Verification items for the finished model (mm, model axes). Face numbers are marked on the shaded views. A direction names the side the tool comes from. Round coordinates to 2 decimals unless told otherwise and drop trailing zeros. Write each loop counter-clockwise with the first axis right and the second up, starting at its lowest first coordinate (ties: lowest second). Pieces come first, ordered by that corner, then holes.
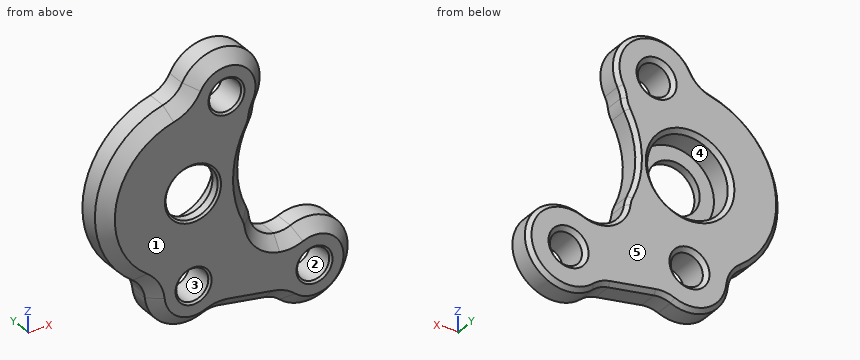
from build123d import *

# Parameters (mm, degrees)
SKETCH1_R           = 9
SKETCH1_R_2         = 4.025
BOSS_EXTRUDE1_DEPTH = 3.5
SKETCH2_R           = 4.1
SKETCH2_R_2         = 1.6
BOSS_EXTRUDE2_DEPTH = 3.5
SKETCH6_R           = 9
CUT_EXTRUDE2_DEPTH  = 17.27435259
CUT_EXTRUDE1_START  = -3.5
SKETCH3_R           = 1.6
CUT_EXTRUDE1_DEPTH  = 3.5
SKETCH4_R           = 1.6
BOSS_EXTRUDE3_DEPTH = 3.5
SKETCH5_R           = 4.025
SKETCH5_R_2         = 2.6
BOSS_EXTRUDE4_DEPTH = 1
FILLET1_R           = 3
FILLET9_R           = 3
CHAMFER_1_SIZE      = 1.2
CHAMFER_2_SIZE      = 0.2
CHAMFER_3_SIZE      = 0.4


with BuildPart() as part:
    # Sketch1 → Boss-Extrude1 (new body)
    with BuildSketch(Plane(origin=(0, 0, 0), x_dir=(1, 0, 0), z_dir=(0, 1, 0))):
        with Locations(Location((0, 0, 0), (0, 0, 270))):
            Circle(SKETCH1_R)
        with Locations(Location((0, 0, 0), (0, 0, 270))):
            Circle(SKETCH1_R_2, mode=Mode.SUBTRACT)
    extrude(amount=BOSS_EXTRUDE1_DEPTH)

    # Sketch2 → Boss-Extrude2 (add)
    # profile 1 of 2: a face of its own
    with BuildSketch(Plane(origin=(0, 3.5, 0), x_dir=(1, 0, 0), z_dir=(0, 1, 0))):
        with Locations((3.343277014, -8.355985807)):
            Circle(SKETCH2_R)
        with Locations((3.343277014, -8.355985807)):
            Circle(SKETCH2_R_2, mode=Mode.SUBTRACT)
    # profile 2 of 2: a face of its own
    with BuildSketch(Plane(origin=(0, 3.5, 0), x_dir=(1, 0, 0), z_dir=(0, 1, 0))):
        with Locations((0.061177946, 8.999792068)):
            Circle(SKETCH2_R)
        with Locations((0.061177946, 8.999792068)):
            Circle(SKETCH2_R_2, mode=Mode.SUBTRACT)
    extrude(amount=-BOSS_EXTRUDE2_DEPTH)

    # Sketch6 → Cut-Extrude2 (cut, through all)
    with BuildSketch(Plane(origin=(0, 0, 0), x_dir=(-1, 0, 0), z_dir=(0, -1, 0))):
        with Locations((-14.2, 0)):
            Circle(SKETCH6_R)
    extrude(amount=-CUT_EXTRUDE2_DEPTH, mode=Mode.SUBTRACT)

    # Sketch3 → Cut-Extrude1 (cut)
    with BuildSketch(Plane(origin=(0, 0, 0), x_dir=(-1, 0, 0), z_dir=(0, -1, 0)).offset(CUT_EXTRUDE1_START)):
        with Locations(Location((-0.061177946, 8.999792068, 0), (0, 0, 270))):
            Circle(SKETCH3_R)
        with Locations(Location((-3.343277014, -8.355985807, 0), (0, 0, 270))):
            Circle(SKETCH3_R)
    extrude(amount=CUT_EXTRUDE1_DEPTH, mode=Mode.SUBTRACT)

    # Sketch4 → Boss-Extrude3 (add)
    with BuildSketch(Plane(origin=(0, 0, 0), x_dir=(-1, 0, 0), z_dir=(0, -1, 0))):
        with BuildLine():
            Line((-2.353733001, 12.398937743), (-8.897987933, 13.432234974))
            ThreePointArc((-8.897987933, 13.432234974), (-16.176141716, 11.544244815), (-9.833757914, 7.505656319))
            Line((-9.833757914, 7.505656319), (-5.813078926, 6.870816065))
            ThreePointArc((-5.813078926, 6.870816065), (-4.964487715, 7.506920922), (-4.04696144, 8.038787415))
            ThreePointArc((-4.04696144, 8.038787415), (-3.883103044, 10.484005175), (-2.353733001, 12.398937743))
        make_face()
        with Locations(Location((-12.126312969, 10.904801994, 0), (0, 0, 90))):
            Circle(SKETCH4_R, mode=Mode.SUBTRACT)
    extrude(amount=-BOSS_EXTRUDE3_DEPTH)

    # Sketch5 → Boss-Extrude4 (add)
    with BuildSketch(Plane(origin=(0, 0, 0), x_dir=(-1, 0, 0), z_dir=(0, -1, 0))):
        with Locations(Location((0, 0, 0), (0, 0, 90))):
            Circle(SKETCH5_R)
        with Locations(Location((0, 0, 0), (0, 0, 90))):
            Circle(SKETCH5_R_2, mode=Mode.SUBTRACT)
    extrude(amount=-BOSS_EXTRUDE4_DEPTH)

    # Fillet1
    # the kernel refuses this fillet: 3 mm, written as the material it adds along each edge
    with BuildSketch(Plane(origin=(-0.71019136, 3.5, 8.97193559), x_dir=(-0.9865858542334134, 0, -0.1632432302624714), z_dir=(0, -1, 0))) as fillet1_piece_1:
        with BuildLine():
            CenterArc((1.782533661, -2.98917289), FILLET1_R, 94.869271374, 48.27534012)
            ThreePointArc((-0.617922081, -1.189780705), (-0.260000299, -0.620318503), (0, 0))
            ThreePointArc((0, 0), (0.763942997, -0.03248133), (1.527885995, 0))
        make_face()
    extrude(amount=3.5)
    with BuildSketch(Plane(origin=(-3.93730186, 3.5, -8.093062095), x_dir=(-0.8588495215516518, 0, 0.5122279759350309), z_dir=(0, -1, 0))) as fillet1_piece_2:
        with BuildLine():
            CenterArc((1.782533661, 2.98917289), FILLET1_R, 216.855388506, 48.27534012)
            ThreePointArc((-0.617922081, 1.189780705), (-0.260000299, 0.620318503), (0, 0))
            ThreePointArc((0, 0), (0.763942997, 0.03248133), (1.527885995, 0))
        make_face()
    extrude(amount=3.5)
    with BuildSketch(Plane(origin=(8.897987933, 0, -13.432234974), x_dir=(-0.9877631090139599, 0, 0.15596166346598195), z_dir=(0, 1, 0))) as fillet1_piece_3:
        with BuildLine():
            CenterArc((1.001412857, -3), FILLET1_R, 90, 32.320518146)
            ThreePointArc((-0.602552177, -0.464788732), (-0.290469322, -0.24640426), (0, 0))
            Line((0, 0), (1.001412857, 0))
        make_face()
    extrude(amount=3.5)
    with BuildSketch(Plane(origin=(2.353733001, 0, -12.398937743), x_dir=(-0.8773738132879287, 0, -0.4798074527939294), z_dir=(0, 1, 0)), Plane(origin=(9.833757914, 0, -7.505656319), x_dir=(0.8773738132879222, 0, 0.47980745279394127), z_dir=(0, 1, 0))) as fillet1_piece_4:
        with BuildLine():
            CenterArc((1.039393717, -2.987053466), FILLET1_R, 95.324882893, 32.320518146)
            Line((-0.792924625, -0.611635715), (0, 0))
            ThreePointArc((0, 0), (0.380492343, -0.017693596), (0.760984685, 0))
        make_face()
    extrude(amount=3.5)
    # the kernel refuses this fillet: 3 mm, written as the material it takes off along each edge
    with BuildSketch(Plane(origin=(7.1, 6.983871428, 5.530822724), x_dir=(-0.6413091964506672, 0, 0.7672825519636162), z_dir=(0, -1, 0))) as fillet1_2_piece_1:
        with BuildLine():
            CenterArc((2.400494629, 2.413903277), FILLET1_R, 201.072777054, 32.502187501)
            ThreePointArc((-0.398878795, 1.335242797), (-0.173557144, 0.675353237), (0, 0))
            ThreePointArc((0, 0), (0.309591521, -0.005326404), (0.619183042, 0))
        make_face()
    extrude(amount=10.467742856, mode=Mode.SUBTRACT)
    with BuildSketch(Plane(origin=(7.1, 8.410224582, -5.530822724), x_dir=(-0.5247859915025788, 0, 0.8512341999254115), z_dir=(0, -1, 0))) as fillet1_2_piece_2:
        with BuildLine():
            CenterArc((2.291438138, 2.982087035), FILLET1_R, 203.232841743, 60.502793026)
            ThreePointArc((-0.465290008, 1.798680965), (-0.279182448, 0.88730199), (0, 0))
            ThreePointArc((0, 0), (0.982044916, 0.053738894), (1.964089833, 0))
        make_face()
    extrude(amount=13.320449164, mode=Mode.SUBTRACT)

    # Fillet9
    fillet9_edges = [part.edges().sort_by_distance(p)[0] for p in [
        (6.702912221, 1.75, 6.005911068),
        (5.813078926, 1.75, -6.870816065),
    ]]
    fillet(fillet9_edges, radius=FILLET9_R)

    # 倒角1
    chamfer_1_edges = [part.edges().sort_by_distance(p)[0] for p in [
        (16.176141716, 0, -11.544244815),
        (5.625860467, 0, -12.915586358),
        (-2.007663811, 0, -12.539551069),
        (5.204560758, 0, 0.286483569),
        (5.220072831, 0, 12.001206989),
        (-8.84326494, 0, 1.672323294),
        (6.564091926, 0, 4.905386326),
        (9.687844205, 0, -7.362609827),
        (8.715099113, 0, -13.523365587),
        (2.49964671, 0, -12.541984235),
        (-4.406035705, 0, -8.239061366),
        (-1.093245074, 0, 9.27901385),
        (8.843752485, 0, -7.349340608),
        (6.238006504, 0, -4.301725459),
        (7.158194759, 0, -6.475494242),
        (6.796639749, 0, 5.998875214),
    ]]
    chamfer(chamfer_1_edges, length=CHAMFER_1_SIZE)

    # 倒角2
    chamfer_2_edges = [part.edges().sort_by_distance(p)[0] for p in [
        (4.706817353, 0, 9.19309855),
        (1.13707684, 0, -7.815544808),
        (12.126312969, 0, -9.304801994),
        (0, 0, 2.6),
    ]]
    chamfer(chamfer_2_edges, length=CHAMFER_2_SIZE)

    # 倒角3
    chamfer_3_edges = [part.edges().sort_by_distance(p)[0] for p in [
        (16.176141716, 3.5, -11.544244815),
        (5.625860467, 3.5, -12.915586358),
        (-2.007663811, 3.5, -12.539551069),
        (5.204560758, 3.5, 0.286483569),
        (-8.84326494, 3.5, 1.672323294),
        (5.220072831, 3.5, 12.001206989),
        (6.238006504, 3.5, -4.301725459),
        (9.687844205, 3.5, -7.362609827),
        (8.715099113, 3.5, -13.523365587),
        (2.49964671, 3.5, -12.541984235),
        (-4.406035705, 3.5, -8.239061366),
        (-1.093245074, 3.5, 9.27901385),
        (8.843752485, 3.5, -7.349340608),
        (6.564091926, 3.5, 4.905386326),
        (7.158194759, 3.5, -6.475494242),
        (6.796639749, 3.5, 5.998875214),
        (4.706817353, 3.5, 9.19309855),
        (1.13707684, 3.5, -7.815544808),
        (0, 3.5, -4.025),
        (12.126312969, 3.5, -9.304801994),
    ]]
    chamfer(chamfer_3_edges, length=CHAMFER_3_SIZE)


solid = part.part
Q1. Tool access check on the marked faces 4 and 5. Record the directions out of +Z, -Z, +X, -X, +Y, -Y that give a thin tool (end or side, any length) a straight path to the whole face; none if there is none.
Recorded:
face 4: +Y
face 5: +Z, -Z, +X, -X, +Y
Q2. Sectioned sample at B-B (z = -10). Give the number of separate pieces and of enclosed holes in the cut face, plus the area to 3 significant figures.
Recorded:
separate pieces: 3
enclosed holes: 0
area: 50.0 mm2
Q3. Release check for a two-part mould opening along Z. For the marked faces 1, 2 and 3 record: released by +Z, released by -Z, zero draft, split by the parting line, or undercut.
Recorded:
face 1: zero draft
face 2: undercut
face 3: undercut
Q4. Depth check by flat-ended pin: P1, Ø2.5, axis at x = 0.06, z = -9, coming from the -Y side. Enter the tip coordinate at first touch or a pass-through.
Recorded:
P1: passes through
Q5. Material ranges on line 1 along Z through (x, y) = (-1, 1.1); line 2 along Z through (x, y) = (0.5, 0.8); line 3 along Z through (x, y) = (4, 0.6) (3 decimals), recorded low to high.
Recorded:
line 1: z = -12.86 to -10.2, -7.8 to -3.9, 3.9 to 9.23
line 2: z = -12.67 to -10.54, -7.46 to -2.55, 2.55 to 10.72
line 3: z = -12.051 to 6.897, 9.815 to 11.794
Q6. Sectioned sample at A-A (z = 0). Enter the section's corners in (x, y) (3 decimals).
Recorded:
outline: (-9, 1.2) - (-7.8, 0) - (-2.8, 0) - (-2.6, 0.2) - (-2.6, 1) - (-4.025, 1) - (-4.025, 3.1) - (-4.425, 3.5) - (-8.6, 3.5) - (-9, 3.1) - close; (2.6, 0.2) - (2.8, 0) - (4, 0) - (5.2, 1.2) - (5.2, 3.1) - (4.8, 3.5) - (4.425, 3.5) - (4.025, 3.1) - (4.025, 1) - (2.6, 1) - close
